Answer from the drawing. Dimensions are ordinates in mm from the lowest x, y and z of the part. A direction names the side the tool comes from. Give positions to 0.01 mm unless a question says otherwise; leave off trailing zeros. Order: outer loops, then holes, each group sorted by start corner. A loop starts at its lowest first (then second) coordinate and runs counter-clockwise, first axis right, second up.
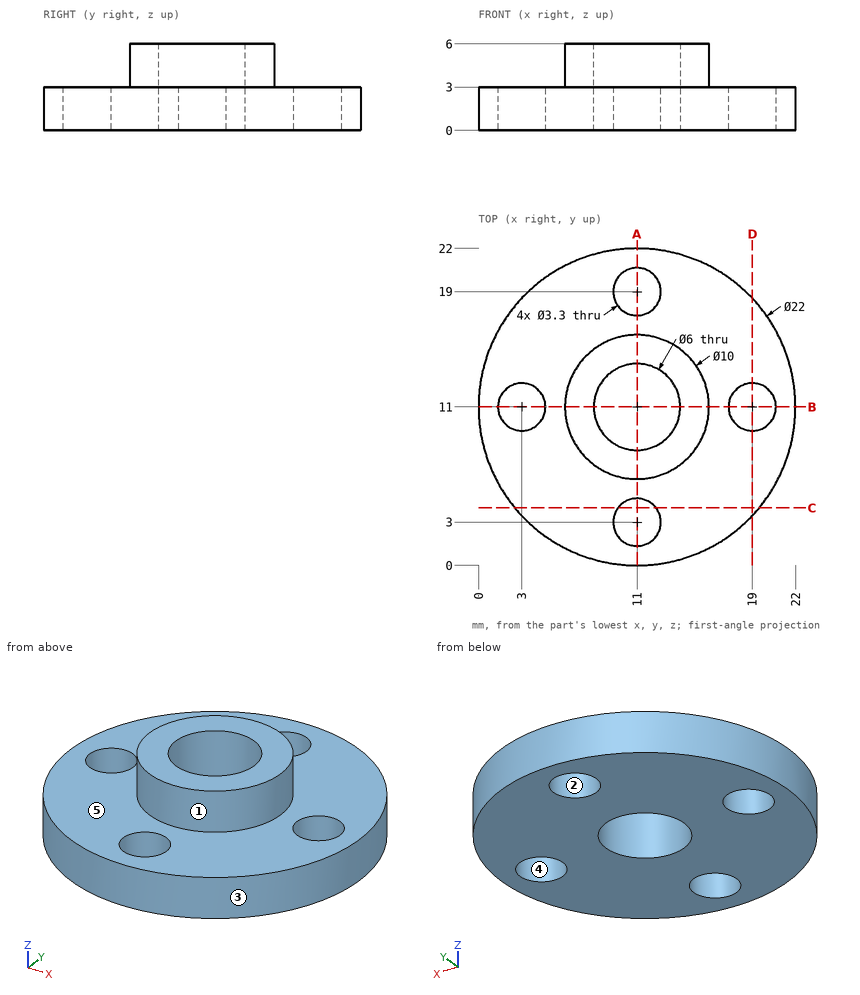
1. The part is cut by section C-C (y = 4). Write down the section's boundary in (x, z).
Findings below:
outline: (2.51, 0) - (9.69, 0) - (9.69, 3) - (2.51, 3) - close; (12.31, 0) - (19.49, 0) - (19.49, 3) - (12.31, 3) - close
2. Straight lines are drawn through the part: probe 1 along Y at (x, z) = (11, 1); probe 2 along Y at (x, z) = (11, 4.65); probe 3 along Z at (x, y) = (12.5, 1.5). For each, find the intervals that lie inside material, in ascending order.
Findings below:
probe 1: y = 0 to 1.35, 4.65 to 8, 14 to 17.35, 20.65 to 22
probe 2: y = 6 to 8, 14 to 16
probe 3: z = 0 to 3
3. Given P1, Ø2, axis at x = 3, y = 11, coming from the -Z side; P2, Ø1, axis at x = 9, y = 17.5, coming from the +Z side; P3, Ø3, axis at y = 14, z = 2.5, coming from the +X side; P4, Ø3, axis at y = 13, z = 2, coming from the -X side, each flat-ended and moving along its own axis, determine where each tip first touches the part or whether it passes through.
Findings below:
P1: passes through
P2: stops at z = 3
P3: stops at x = 21.9
P4: stops at x = 0.01
4. The part is cut by section A-A (x = 11). Write down the section's boundary in (y, z), then the cut area to 3 significant figures.
Findings below:
outline: (0, 0) - (1.35, 0) - (1.35, 3) - (0, 3) - close; (4.65, 0) - (8, 0) - (8, 6) - (6, 6) - (6, 3) - (4.65, 3) - close; (14, 0) - (17.35, 0) - (17.35, 3) - (16, 3) - (16, 6) - (14, 6) - close; (20.65, 0) - (22, 0) - (22, 3) - (20.65, 3) - close
area: 40.2 mm2
5. The mould has two halves that part along Y. Classify the marked faces 3, 4 and 5: pulls with the +Y half, pulls with the -Y half, needs draft (parallel to the pull), parting line crosses it, or undercut.
Findings below:
face 3: parting line crosses it
face 4: undercut
face 5: needs draft
6. The part is cut by section D-D (x = 19). Write down the section's boundary in (y, z), then the cut area to 3 significant figures.
Findings below:
outline: (3.45, 0) - (9.35, 0) - (9.35, 3) - (3.45, 3) - close; (12.65, 0) - (18.55, 0) - (18.55, 3) - (12.65, 3) - close
area: 35.4 mm2
7. Which of the six approach directions +Z, -Z, +X, -X, +Y, -Y give full straight-line access (tool end or side, diameter ignored) to the marked faces 1 and 2?
Findings below:
face 1: +Z
face 2: +Z, -Z
